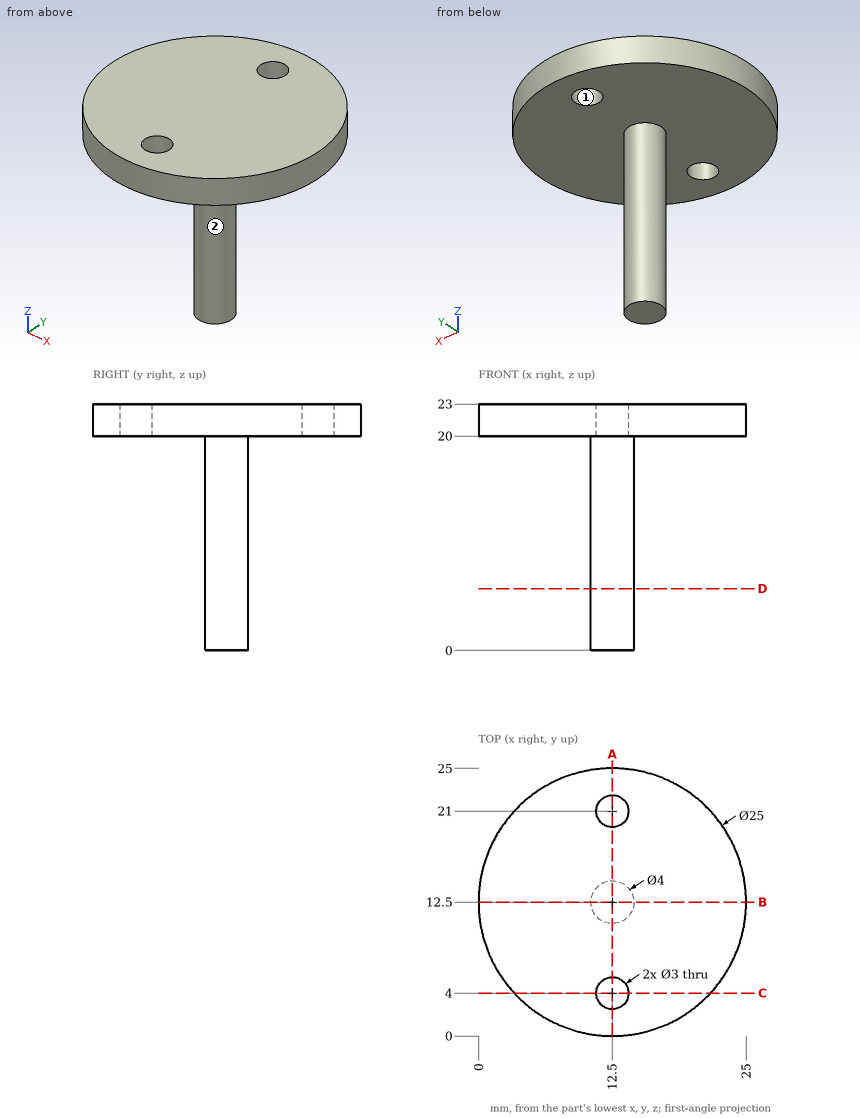
Geometry check sheet. Reference: drawing and pictorial views, mm from the part's lowest x, y, z. A direction names the side the tool comes from. Round coordinates to 2 decimals unless told otherwise and drop trailing zeros. Write each loop counter-clockwise with the first axis right and the second up, starting at its lowest first coordinate (ties: lowest second). Pieces come first, ordered by that corner, then holes.
1. Gauge pin test, flat ends, axial feed: P1, Ø1, axis at x = 13, y = 9, coming from the -Z side; P2, Ø3.5, axis at x = 12.5, y = 21, coming from the +Z side; P3, Ø12, axis at y = 15.5, z = 3.5, coming from the -X side; P4, Ø10, axis at x = 8.5, z = 10, coming from the +Y side. Record the tip position at first contact, or that the pin passes through.
2. Section check C-C on y = 4. Enter the section's corners in (x, z), plus the area to 3 significant figures.
3. Section check D-D on z = 5.75. Enter the section's corners in (x, y), plus the area to 3 significant figures.
4. Access from +Z, -Z, +X, -X, +Y, -Y to the whole of each face (thin tool, end or side, straight path). Record for the marked faces 1 and 2.
5. Scan lines: L1, parallel to Y at x = 12.5, z = 22; L2, parallel to Z at x = 22.75, y = 12.75; L3, parallel to X at y = 12, z = 15.5. Record each from-to range of solid material in increasing order.
6. Section check A-A on x = 12.5. Enter the section's corners in (y, z).
7. Section check B-B on y = 12.5. Enter the section's corners in (x, z).
Answer:
1. P1: stops at z = 20
1. P2: stops at z = 23
1. P3: stops at x = 10.5
1. P4: stops at y = 14.5
2. outline: (3.33, 20) - (11, 20) - (11, 23) - (3.33, 23) - close; (14, 20) - (21.67, 20) - (21.67, 23) - (14, 23) - close
2. area: 46.0 mm2
3. outline: circle Ø4 at (12.5, 12.5)
3. area: 12.6 mm2
4. face 1: +Z, -Z
4. face 2: -Z
5. L1: y = 0 to 2.5, 5.5 to 19.5, 22.5 to 25
5. L2: z = 20 to 23
5. L3: x = 10.56 to 14.44
6. outline: (0, 20) - (2.5, 20) - (2.5, 23) - (0, 23) - close; (5.5, 20) - (10.5, 20) - (10.5, 0) - (14.5, 0) - (14.5, 20) - (19.5, 20) - (19.5, 23) - (5.5, 23) - close; (22.5, 20) - (25, 20) - (25, 23) - (22.5, 23) - close
7. outline: (0, 20) - (10.5, 20) - (10.5, 0) - (14.5, 0) - (14.5, 20) - (25, 20) - (25, 23) - (0, 23) - close
